Autodesk Fusion 360 part; units mm, degrees
sketch "Sketch1" plane through (0, 0, 0) normal (0, 0, 1) x (1, 0, 0)
  line L0 (120, 20) -> (-120, 20)
  line L1 (-120, 20) -> (-120, -20)
  line L2 (-120, -20) -> (120, -20)
  line L3 (120, -20) -> (120, 20)
  line L4 (120, 20) -> (-120, -20) construction
  line L5 (-120, 20) -> (120, -20) construction
  dimension "d1" = 240
  dimension "d2" = 40
extrude "Extrude1" add sketch "Sketch1" along normal blind 5
sketch "Sketch2" plane through (0, 0, 5) normal (0, 0, 1) x (-1, 0, 0)
  line L0 (-120, 20) -> (-120, -20)
  line L1 (120, -20) -> (120, 20)
  line L2 (120, 20) -> (-120, 20)
  line L3 (120, -20) -> (-120, -20)
  line L4 (-120, -20) -> (-120, -16)
  line L5 (-120, -16) -> (120, -16)
  line L6 (120, -16) -> (120, -20)
  line L7 (-120, -20) -> (120, -20)
  dimension "d7" = 4
extrude "Extrude3" add sketch "Sketch2" along normal blind 30 contours L0 L1 L3 L4 L5 L6 L7
sketch "Sketch3" plane through (0, 20, 0) normal (0, 1, 0) x (-1, 0, 0)
  line L0 (-120, 0) -> (120, 0)
  line L1 (120, 0) -> (120, 35)
  line L2 (120, 35) -> (-120, 35)
  line L3 (-120, 35) -> (-120, 0)
  line L4 (0, 35) -> (0, 0) construction
  line L5 (20.55, 35) -> (20.55, 0) construction
  line L6 (61.65, 35) -> (61.65, 0) construction
  line L7 (102.75, 35) -> (102.75, 0) construction
  line L8 (-20.55, 35) -> (-20.55, 0) construction
  line L9 (-61.65, 35) -> (-61.65, 0) construction
  line L10 (-102.75, 35) -> (-102.75, 0) construction
  line L11 (120, 17.5) -> (-120, 17.5) construction
  line L12 (27.95, 17.5) -> (24.25, 23.9086)
  line L13 (24.25, 23.9086) -> (16.85, 23.9086)
  line L14 (16.85, 23.9086) -> (13.15, 17.5)
  line L15 (13.15, 17.5) -> (16.85, 11.0914)
  line L16 (16.85, 11.0914) -> (24.25, 11.0914)
  line L17 (24.25, 11.0914) -> (27.95, 17.5)
  line L18 (-13.15, 17.5) -> (-16.85, 23.9086)
  line L19 (-16.85, 23.9086) -> (-24.25, 23.9086)
  line L20 (-24.25, 23.9086) -> (-27.95, 17.5)
  line L21 (-27.95, 17.5) -> (-24.25, 11.0914)
  line L22 (-24.25, 11.0914) -> (-16.85, 11.0914)
  line L23 (-16.85, 11.0914) -> (-13.15, 17.5)
  line L24 (-95.35, 17.5) -> (-99.05, 23.9086)
  line L25 (-99.05, 23.9086) -> (-106.45, 23.9086)
  line L26 (-106.45, 23.9086) -> (-110.15, 17.5)
  line L27 (-110.15, 17.5) -> (-106.45, 11.0914)
  line L28 (-106.45, 11.0914) -> (-99.05, 11.0914)
  line L29 (-99.05, 11.0914) -> (-95.35, 17.5)
  line L30 (95.35, 17.5) -> (99.05, 11.0914)
  line L31 (99.05, 11.0914) -> (106.45, 11.0914)
  line L32 (106.45, 11.0914) -> (110.15, 17.5)
  line L33 (110.15, 17.5) -> (106.45, 23.9086)
  line L34 (106.45, 23.9086) -> (99.05, 23.9086)
  line L35 (99.05, 23.9086) -> (95.35, 17.5)
  point P0 (20.55, 17.5)
  point P1 (-20.55, 17.5)
  point P2 (-102.75, 17.5)
  point P3 (102.75, 17.5)
  dimension "d10" = 20.55
  dimension "d11" = 41.1
  dimension "d12" = 41.1
  dimension "d13" = 41.1
  dimension "d14" = 41.1
  dimension "d15" = 20.55
  dimension "d16" = 7.4
  dimension "d17" = 7.4
  dimension "d18" = 7.4
  dimension "d19" = 7.4
extrude "Extrude4" add sketch "Sketch3" along normal blind 10 contours L12 L13 L14 L15 L16 L17 | L18 L19 L20 L21 L22 L23 | L24 L25 L26 L27 L28 L29 | L30 L31 L32 L33 L34 L35
extrude "Extrude8" cut 1 faces at (-40, -20, 1.6667) along direction (0, 1, 0) up to surface (36 mm away)
chamfer "Chamfer15" distance 1.5 angle 45 24 edges at (102.75, 30, 23.9086) (108.3, 30, 20.7043) (108.3, 30, 14.2957) (97.2, 30, 20.7043) (97.2, 30, 14.2957) (102.75, 30, 11.0914) (20.55, 30, 23.9086) (26.1, 30, 20.7043) (26.1, 30, 14.2957) (15, 30, 20.7043) (15, 30, 14.2957) (20.55, 30, 11.0914) (-20.55, 30, 23.9086) (-15, 30, 20.7043) (-15, 30, 14.2957) (-26.1, 30, 20.7043) (-26.1, 30, 14.2957) (-20.55, 30, 11.0914) (-102.75, 30, 23.9086) (-97.2, 30, 20.7043) (-97.2, 30, 14.2957) (-108.3, 30, 20.7043) (-108.3, 30, 14.2957) (-102.75, 30, 11.0914)
fillet "Fillet3" radius 1.5 24 edges at (99.05, 24.25, 23.9086) (110.15, 24.25, 17.5) (106.45, 24.25, 23.9086) (106.45, 24.25, 11.0914) (16.85, 24.25, 23.9086) (24.25, 24.25, 23.9086) (27.95, 24.25, 17.5) (24.25, 24.25, 11.0914) (-24.25, 24.25, 23.9086) (-16.85, 24.25, 23.9086) (-13.15, 24.25, 17.5) (-16.85, 24.25, 11.0914) (-106.45, 24.25, 23.9086) (-99.05, 24.25, 23.9086) (-95.35, 24.25, 17.5) (-99.05, 24.25, 11.0914) (-110.15, 24.25, 17.5) (-106.45, 24.25, 11.0914) (-27.95, 24.25, 17.5) (-24.25, 24.25, 11.0914) (13.15, 24.25, 17.5) (16.85, 24.25, 11.0914) (95.35, 24.25, 17.5) (99.05, 24.25, 11.0914)
equation "d22 = ( 240 / 6 ) * 1 mm"
Design review of the part built by this model. Coordinates are the model's own, in mm. A direction names the side the tool comes from. Coordinates: 2 decimals unless noted, no trailing zeros. Order: outer loops, then holes, each group sorted by start corner. A loop starts at its lowest first (then second) coordinate and runs counter-clockwise, first axis right, second up.
1) Take a section at A-A, the plane x = -102. Give the boundary of the cut face in (y, z), and give its area (3 significant figures).
2) For faces 1 (the flat face through (108.32, 24.19, 14.33)), 2 (the flat face through (-15.684, 29.261, 14.632)), 3 (the flat face through (25.47, 29.26, 20.28)), 4 (the flat face through (-103, 24, 23.909)), list the 3-axis set-ups (+Z, -Z, +X, -X, +Y, -Y) from which the entire face can be reached by the end or side of a thin tool; tool diameter is ignored.
3) Take a section at C-C, the plane z = 6. Give the boundary of the cut face in (x, y).
4) Take a section at D-D, the plane x = 4.5. Give the boundary of the cut face in (y, z), and give its area (3 significant figures).
5) Take a section at B-B, the plane y = 26.25. State how many separate pieces and enclosed holes the cut face has, and give its area (3 significant figures).
6) Mouldability with a two-part tool opening along X and no side actions: class faces 5 (the flat face through (-15.63, 29.26, 20.28)), 6 (the flat face through (-107.616, 29.261, 20.368)), 7 (the flat face through (2, 16, 17)) as +X half, -X half, draft (parallel to the pull), parting line (faces both ways), or undercut.
7) Wall thickness on line 1 along X through (y, z) = (26, 14.5); line 2 along X through (y, z) = (23.75, 16.5); line 3 along Y through (x, z) = (-55, 3.5): over which ranges is each line inside the solid? List them lowest first.
8) Clearance check with flat-ended pins moving along their axes: pin 1 (4.5 mm diameter, centred on x = -103.5, y = 22.5, fed in from -Z); pin 2 (1.5 mm diameter, centred on x = -6, z = 17.5, fed in from +Y); pin 3 (3 mm diameter, centred on x = -103, y = 25, fed in from +Z). State where each tip first meets the part, or that it passes through.
Returned:
1. outline: (16, 0) - (20, 0) - (20, 11.09) - (28.5, 11.09) - (30, 12.59) - (30, 22.41) - (28.5, 23.91) - (20, 23.91) - (20, 35) - (16, 35) - close
1. area: 266 mm2
2. face 1: -Z, +X, +Y
2. face 2: -Z, +Y
2. face 3: +Z, +Y
2. face 4: +Z, +X, -X, +Y
3. outline: (-120, 16) - (120, 16) - (120, 20) - (-120, 20) - close
4. outline: (16, 0) - (20, 0) - (20, 35) - (16, 35) - close
4. area: 140 mm2
5. separate pieces: 4
5. enclosed holes: 0
5. area: 566 mm2
6. face 5: undercut
6. face 6: -X half
6. face 7: draft
7. line 1: x = -108.42 to -97.08, -26.22 to -14.88, 14.88 to 26.22, 97.08 to 108.42
7. line 2: x = -109.57 to -95.93, -27.37 to -13.73, 13.73 to 27.37, 95.93 to 109.57
7. line 3: y = 16 to 20
8. pin 1: stops at z = 11.09
8. pin 2: stops at y = 20
8. pin 3: stops at z = 23.91
